```python
from build123d import *

# Parameters (mm, degrees)
PAD_DEPTH        = 13
HOLE_D           = 6.6
HOLE_DEPTH       = 25
HOLE_CBORE_D     = 11
HOLE_CBORE_DEPTH = 6.4
FILLET_R         = 2
FILLET001_R      = 2
FILLET002_R      = 2
FILLET003_R      = 2


with BuildPart() as part:
    # Sketch → Pad (new body)
    with BuildSketch(Plane.XY):
        with BuildLine():
            ThreePointArc((25, 25), (0, 35.355339), (-25, 25))
            Line((-25, -27.95085), (-25, 25))
            ThreePointArc((-25, -27.95085), (0, -37.5), (25, -27.95085))
            Line((25, 25), (25, -27.95085))
        make_face()
        with BuildLine():
            ThreePointArc((-19.834345, -19.834345), (0, -28.05), (19.834345, -19.834345))
            ThreePointArc((19.834345, -19.834345), (19.834345, -15.520994), (15.520994, -15.520994))
            ThreePointArc((-15.520994, -15.520994), (0, -21.95), (15.520994, -15.520994))
            ThreePointArc((-15.520994, -15.520994), (-19.834345, -15.520994), (-19.834345, -19.834345))
        make_face(mode=Mode.SUBTRACT)
        with BuildLine():
            ThreePointArc((-19.834345, 19.834345), (-19.834345, 15.520994), (-15.520994, 15.520994))
            ThreePointArc((15.521007, 15.52098), (1e-05, 21.95), (-15.520994, 15.520994))
            ThreePointArc((15.521007, 15.52098), (19.834352, 15.521), (19.834346, 19.834345))
            ThreePointArc((19.834346, 19.834345), (0, 28.05), (-19.834345, 19.834345))
        make_face(mode=Mode.SUBTRACT)
    extrude(amount=PAD_DEPTH)

    # Hole
    with Locations(Plane(origin=(0, 0, 0), x_dir=(1, 0, 0), z_dir=(0, 0, -1))):
        with Locations((0, 0), (-12.5, 0), (12.5, 0)):
            CounterBoreHole(HOLE_D / 2, HOLE_CBORE_D / 2, HOLE_CBORE_DEPTH, depth=HOLE_DEPTH)

    # Fillet
    fillet_edges = [part.edges().sort_by_distance(p)[0] for p in [
        (-25, -1.475425, 13),
    ]]
    fillet(fillet_edges, radius=FILLET_R)

    # Fillet001
    fillet001_edges = [part.edges().sort_by_distance(p)[0] for p in [
        (1.301993, -37.477391, 13),
    ]]
    fillet(fillet001_edges, radius=FILLET001_R)

    # Fillet002
    fillet002_edges = [part.edges().sort_by_distance(p)[0] for p in [
        (1.362703, 35.329068, 13),
    ]]
    fillet(fillet002_edges, radius=FILLET002_R)

    # Fillet003
    fillet003_edges = [part.edges().sort_by_distance(p)[0] for p in [
        (25, -1.561492, 13),
    ]]
    fillet(fillet003_edges, radius=FILLET003_R)


solid = part.part
```
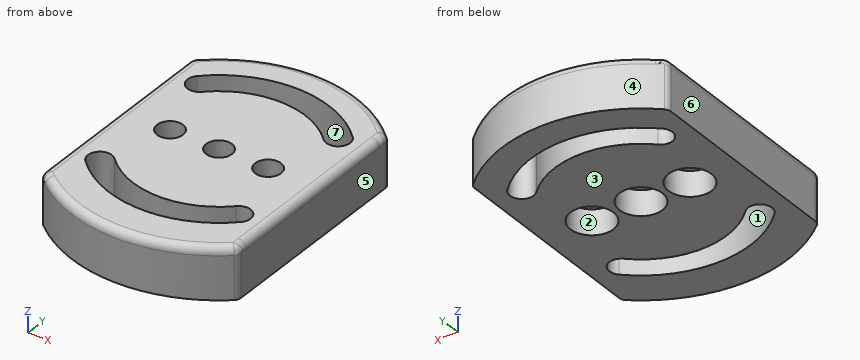
Input: part model. Units: mm. Frame: model coordinates. Face numbers are marked on the shaded views. A direction names the side the tool comes from. Coordinates: 2 decimals unless noted, no trailing zeros. Loops run counter-clockwise (first coordinate to the right, second up) from the corner with the lowest first, then second, coordinate; pieces in that order, holes last. Notation, with made-up numbers: (-17.75, -15.75) - (28.25, -15.75) arc R9 cw to (28.25, -5.75) - close; hole circle Ø10 at (85, 13). An arc over 180 degrees is marked (long way). Answer in a Markdown table with one row per item.
(1) Cut plane C-C on y = 17. Output: boundary loops of the cut face in (x, z).
Model answer:
| item | result |
|---|---|
| outline | (-25, 0) - (-20.65, 0) - (-20.65, 13) - (-23, 13) arc R2 ccw to (-25, 11) - close; (-13.89, 0) - (13.89, 0) - (13.89, 13) - (-13.89, 13) - close; (20.65, 0) - (25, 0) - (25, 11) arc R2 ccw to (23, 13) - (20.65, 13) - close |
(2) Cut plane D-D on x = -12.5. Count the separate pieces of the cut face and the enclosed holes in it, plus the area to 3 significant figures.
Model answer:
| item | result |
|---|---|
| separate pieces | 4 |
| enclosed holes | 0 |
| area | 590 mm² |
(3) Set-up query: the marked faces 1, 2 and 3. Return all of +Z, -Z, +X, -X, +Y, -Y with unobstructed straight access to the full face (end or side cutting, diameter ignored); none if empty.
Model answer:
| item | result |
|---|---|
| face 1 | +Z, -Z |
| face 2 | -Z |
| face 3 | -Z, +X, -X, +Y, -Y |
(4) Pin query (flat end, axial travel): P1, Ø12, axis at x = 14.5, y = -1.5, coming from the -Z side; P2, Ø8.5, axis at x = 12.5, y = 0, coming from the -Z side. Return the tip coordinate at first contact, or that it passes through.
Model answer:
| item | result |
|---|---|
| P1 | stops at z = 0 |
| P2 | stops at z = 6.4 |
(5) Cut plane A-A on x = 0. Output: boundary loops of the cut face in (y, z), plus the area to 3 significant figures.
Model answer:
| item | result |
|---|---|
| outline | (-37.5, 0) - (-28.05, 0) - (-28.05, 13) - (-35.5, 13) arc R2 ccw to (-37.5, 11) - close; (-21.95, 0) - (-5.5, 0) - (-5.5, 6.4) - (-3.3, 6.4) - (-3.3, 13) - (-21.95, 13) - close; (3.3, 6.4) - (5.5, 6.4) - (5.5, 0) - (21.95, 0) - (21.95, 13) - (3.3, 13) - close; (28.05, 0) - (35.36, 0) - (35.36, 11) arc R2 ccw to (33.36, 13) - (28.05, 13) - close |
| area | 673 mm² |
(6) Mould query, pull axis X, two halves, no side actions, for the marked faces 4, 5, 6 and 7. Classes: pulls with the +X half, pulls with the -X half, needs draft (parallel to the pull), parting line crosses it, or undercut.
Model answer:
| item | result |
|---|---|
| face 4 | parting line crosses it |
| face 5 | pulls with the +X half |
| face 6 | pulls with the -X half |
| face 7 | undercut |
(7) Cut plane B-B on z = 5. Output: boundary loops of the cut face in (x, y), plus the area to 3 significant figures.
Model answer:
| item | result |
|---|---|
| outline | (-25, -27.04) arc R2 ccw to (-24.3, -28.57) arc R37.5 ccw to (24.3, -28.57) arc R2 ccw to (25, -27.04) - (25, 24.16) arc R2 ccw to (24.38, 25.61) arc R35.36 ccw to (-24.38, 25.61) arc R2 ccw to (-25, 24.16) - close; hole (-19.83, -19.83) arc R28.05 ccw to (19.83, -19.83) arc R3.05 ccw to (15.52, -15.52) arc R21.95 cw to (-15.52, -15.52) arc R3.05 ccw to start; hole (-19.83, 19.83) arc R3.05 ccw to (-15.52, 15.52) arc R21.95 cw to (15.52, 15.52) arc R3.05 ccw to (19.83, 19.83) arc R28.05 ccw to start; hole circle Ø11 at (-12.5, 0); hole circle Ø11 at (0, 0); hole circle Ø11 at (12.5, 0) |
| area | 2,510 mm² |
(8) Material intervals for L1, parallel to Y at x = 0, z = 9.5; L2, parallel to Y at x = -12, z = 5.75; L3, parallel to Y at x = -19, z = 8.25, sorted ascending. Write a range as from..to.
Model answer:
| item | result |
|---|---|
| L1 | y = -37.5..-28.05, -21.95..-3.3, 3.3..21.95, 28.05..35.36 |
| L2 | y = -35.53..-25.35, -18.38..-5.48, 5.48..18.38, 25.35..33.26 |
| L3 | y = -32.33..-20.63, -14.93..14.93, 20.63..29.82 |
